Job drawing, mm, ordinate dimensions from the low corner. One solid piece. A direction names the side the tool comes from. Coordinates: 2 decimals unless noted, no trailing zeros. Loops run counter-clockwise (first coordinate to the right, second up) from the corner with the lowest first, then second, coordinate; pieces in that order, holes last. Notation, with made-up numbers: (26, 45) - (53, 45) arc R26 ccw to (53, 78) - close; hole circle Ø11 at (23, 14.5). An arc over 180 degrees is marked (long way). Use a Markdown table: item, result. Add a question column.
1. Band-saw the part on A-A, the plane x = 203.2. Give the cut face in (y, z), plus the area to 3 significant figures.
2. Pull direction X, two halves, no side cores. Call the marked faces 3, 4 and 5: pulls with the +X half, pulls with the -X half, needs draft (parallel to the pull), parting line crosses it, or undercut.
3. Wall check: probe 1 along Y at (x, z) = (185, 95.5); probe 2 along Y at (x, z) = (203.2, 8.75). Give the ranges that are in metal, low to high. Write a range as [from, to].
4. 3-axis set-ups, long thin cutter, end or side, ignore diameter. For the marked faces 1 and 2: which of +Z, -Z, +X, -X, +Y, -Y reach the whole face in a straight line?
5. Band-saw the part on B-B, the plane z = 96. Give the cut face in (x, y).
6. Band-saw the part on D-D, the plane x = 327. Give the cut face in (y, z), plus the area to 3 significant figures.
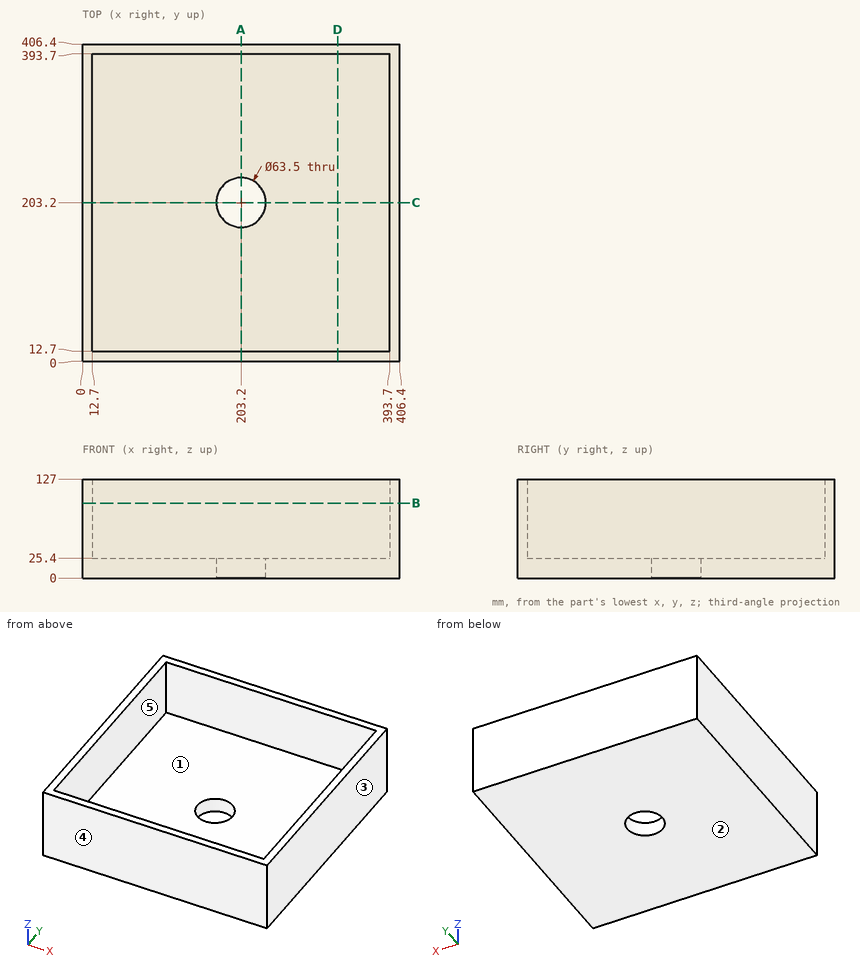
Geometry check:
| question | item | result |
|---|---|---|
| 1 | outline | (0, 0) - (171.45, 0) - (171.45, 25.4) - (12.7, 25.4) - (12.7, 127) - (0, 127) - close; (234.95, 0) - (406.4, 0) - (406.4, 127) - (393.7, 127) - (393.7, 25.4) - (234.95, 25.4) - close |
| 1 | area | 11,300 mm^2 |
| 2 | face 3 | pulls with the +X half |
| 2 | face 4 | needs draft |
| 2 | face 5 | undercut |
| 3 | probe 1 | y = [0, 12.7], [393.7, 406.4] |
| 3 | probe 2 | y = [0, 171.45], [234.95, 406.4] |
| 4 | face 1 | +Z |
| 4 | face 2 | -Z, +X, -X, +Y, -Y |
| 5 | outline | (0, 0) - (406.4, 0) - (406.4, 406.4) - (0, 406.4) - close; hole (12.7, 12.7) - (393.7, 12.7) - (393.7, 393.7) - (12.7, 393.7) - close |
| 6 | outline | (0, 0) - (406.4, 0) - (406.4, 127) - (393.7, 127) - (393.7, 25.4) - (12.7, 25.4) - (12.7, 127) - (0, 127) - close |
| 6 | area | 12,900 mm^2 |
